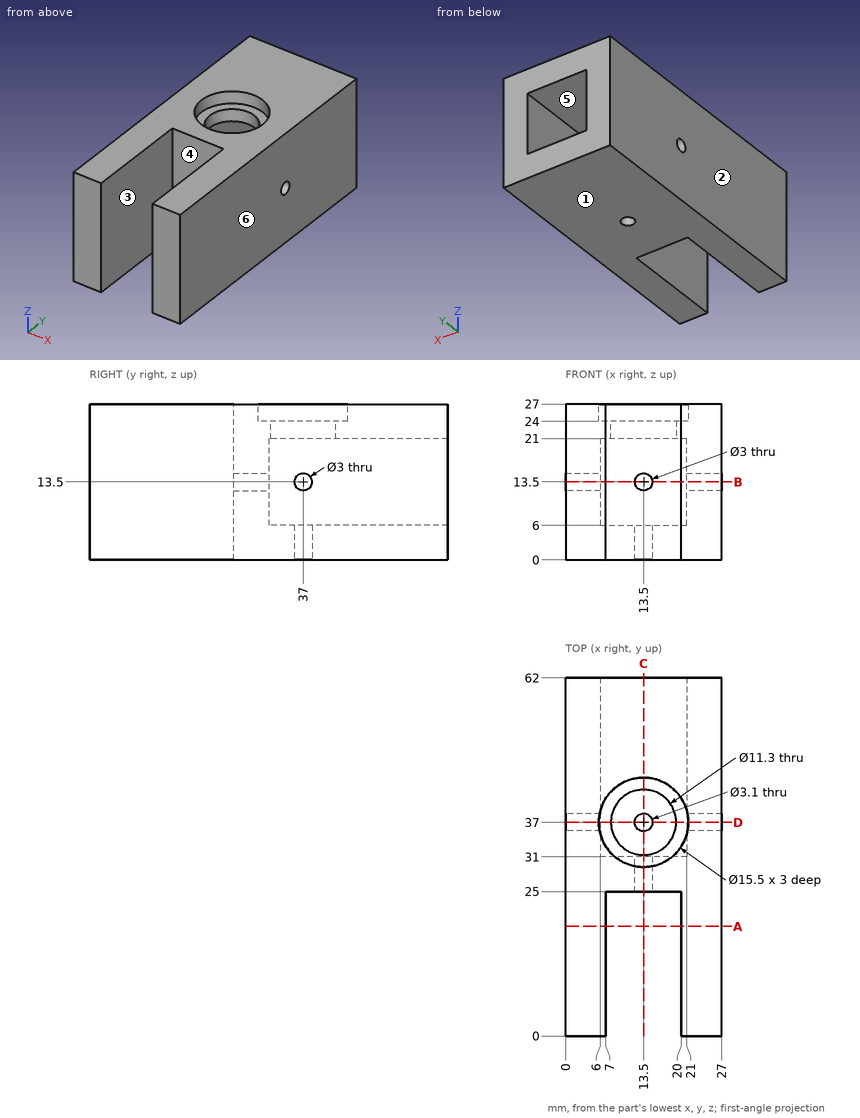
Geometry: see drawing. Coordinates: mm, zero at the bounding-box minimum. A direction names the side the tool comes from. Round coordinates to 2 decimals unless told otherwise and drop trailing zeros. Loops run counter-clockwise (first coordinate to the right, second up) from the corner with the lowest first, then second, coordinate; pieces in that order, holes last. Notation, with made-up numbers: (-6.75, 59) - (29.25, 59) arc R21 ccw to (29.25, 64) - close; hole circle Ø2 at (-34.5, -39.75). An arc over 180 degrees is marked (long way). Write item = value, one per line. Start each with the question number.
(1) Pin query (flat end, axial travel): pin 1 (2.5 mm diameter, centred on y = 37, z = 13.5, fed in from -X); pin 2 (9 mm diameter, centred on x = 13.5, y = 37, fed in from +Z); pin 3 (8 mm diameter, centred on x = 16, y = 35.5, fed in from +Z). Return the tip coordinate at first contact, or that it passes through.
(2) Section query D-D, the plane y = 37. Output: boundary loops of the cut face in (x, z), plus the area to 3 significant figures.
(3) Ray query, line 1 along Z through (x, y) = (14.25, 52); line 2 along X through (y, z) = (16, 16.75); line 3 along X through (y, z) = (37, 25.75). Return the intervals inside material, ascending. Write a range as from..to.
(4) Section query A-A, the plane y = 19. Output: boundary loops of the cut face in (x, z), plus the area to 3 significant figures.
(5) Section query B-B, the plane z = 13.5. Output: boundary loops of the cut face in (x, y).
(6) Pull-direction query (X, two-part tool) for the marked faces 1, 2 and 3; classes: +X half, -X half, draft (parallel to the pull), parting line (faces both ways), or undercut.
(7) Set-up query: the marked faces 4, 5 and 6. Return all of +Z, -Z, +X, -X, +Y, -Y with unobstructed straight access to the full face (end or side cutting, diameter ignored); none if empty.
(8) Section query C-C, the plane x = 13.5. Output: boundary loops of the cut face in (y, z), plus the area to 3 significant figures.
Conclusion:
q1.pin_1 = through
q1.pin_2 = 6
q1.pin_3 = 24
q2.outline = (0, 0) - (11.95, 0) - (11.95, 6) - (6, 6) - (6, 12) - (0, 12) - close; (0, 15) - (6, 15) - (6, 21) - (7.85, 21) - (7.85, 24) - (5.75, 24) - (5.75, 27) - (0, 27) - close; (15.05, 0) - (27, 0) - (27, 12) - (21, 12) - (21, 6) - (15.05, 6) - close; (19.15, 21) - (21, 21) - (21, 15) - (27, 15) - (27, 27) - (21.25, 27) - (21.25, 24) - (19.15, 24) - close
q2.area = 369 mm2
q3.line_1 = 0..6, 21..27
q3.line_2 = 0..7, 20..27
q3.line_3 = 0..5.75, 21.25..27
q4.outline = (0, 0) - (7, 0) - (7, 27) - (0, 27) - close; (20, 0) - (27, 0) - (27, 27) - (20, 27) - close
q4.area = 378 mm2
q5.outline = (0, 0) - (7, 0) - (7, 25) - (12, 25) - (12, 31) - (6, 31) - (6, 35.5) - (0, 35.5) - close; (0, 38.5) - (6, 38.5) - (6, 62) - (0, 62) - close; (15, 25) - (20, 25) - (20, 0) - (27, 0) - (27, 35.5) - (21, 35.5) - (21, 31) - (15, 31) - close; (21, 38.5) - (27, 38.5) - (27, 62) - (21, 62) - close
q6.face_1 = draft
q6.face_2 = -X half
q6.face_3 = undercut
q7.face_4 = +Z, -Z, -Y
q7.face_5 = +Y
q7.face_6 = +Z, -Z, +X, +Y, -Y
q8.outline = (25, 0) - (35.45, 0) - (35.45, 6) - (31, 6) - (31, 12) - (25, 12) - close; (25, 15) - (31, 15) - (31, 21) - (31.35, 21) - (31.35, 24) - (29.25, 24) - (29.25, 27) - (25, 27) - close; (38.55, 0) - (62, 0) - (62, 6) - (38.55, 6) - close; (42.65, 21) - (62, 21) - (62, 27) - (44.75, 27) - (44.75, 24) - (42.65, 24) - close
q8.area = 417 mm2
